```python
from build123d import *

# Parameters (mm, degrees)
F0_W      = 100.4
F0_H      = 7.3
F1_DEPTH  = 1.7
F2_R      = 1.5
F3_DEPTH  = 1.701
F4_W      = 10
F4_H      = 7.3
F5_DEPTH  = 2
F7_W      = 0.2
F7_H      = 7.3
F8_DEPTH  = 0.3
F9_W      = 0.2
F9_H      = 7.3
F10_DEPTH = 0.3


with BuildPart() as f1:
    # F0 (on Front) → F1 (new body)
    with BuildSketch(Plane.XZ):
        Rectangle(F0_W, F0_H)
    extrude(amount=F1_DEPTH)

    # F2 (on face) → F3 (cut, through all)
    with BuildSketch(Plane.XZ.offset(1.7)):
        with Locations((-28.75, -1.35)):
            Circle(F2_R)
        with Locations((-22.35, -1.35)):
            Circle(F2_R)
        with Locations((-15.95, -1.35)):
            Circle(F2_R)
        with Locations((-9.55, -1.35)):
            Circle(F2_R)
        with Locations((-3.15, -1.35)):
            Circle(F2_R)
        with Locations((3.25, -1.35)):
            Circle(F2_R)
        with Locations((9.65, -1.35)):
            Circle(F2_R)
        with Locations((16.05, -1.35)):
            Circle(F2_R)
        with Locations((22.45, -1.35)):
            Circle(F2_R)
        with Locations((28.85, -1.35)):
            Circle(F2_R)
    extrude(amount=-F3_DEPTH, mode=Mode.SUBTRACT)

    # F4 (on face) → F5 (join)
    with BuildSketch(Plane(origin=(0, 0, 0), x_dir=(-1, 0, 0), z_dir=(0, 1, 0))):
        with Locations((-45.2, 0)):
            Rectangle(F4_W, F4_H)
    extrude(amount=F5_DEPTH)

    # F7 (on face) → F8 (cut)
    with BuildSketch(Plane(origin=(0, 0, 0), x_dir=(-1, 0, 0), z_dir=(0, 1, 0))):
        with Locations((40.1, 0)):
            Rectangle(F7_W, F7_H)
    extrude(amount=-F8_DEPTH, mode=Mode.SUBTRACT)

    # F9 (on face) → F10 (cut)
    with BuildSketch(Plane(origin=(0, 0, 0), x_dir=(-1, 0, 0), z_dir=(0, 1, 0))):
        with Locations((43.1, 0)):
            Rectangle(F9_W, F9_H)
    extrude(amount=-F10_DEPTH, mode=Mode.SUBTRACT)


solid = f1.part
```
Model file for the job. Use its own axes, mm. A direction names the side the tool comes from. Give positions to 0.01 mm unless a question says otherwise; leave off trailing zeros. Loops run counter-clockwise (first coordinate to the right, second up) from the corner with the lowest first, then second, coordinate; pieces in that order, holes last. Notation, with made-up numbers: (17.25, 15) -> (53.25, 15) arc R15 cw to (53.25, 20) -> close; hole circle Ø10 at (44.25, -17). An arc over 180 degrees is marked (long way). Write each question's results on one line, items separated by ' | '.
(1) Cut at A-A on x = -9.55. List the corners of the cut face in (y, z), and give its area (3 significant figures).
Geometry results:
outline: (-1.7, -3.65) -> (0, -3.65) -> (0, -2.85) -> (-1.7, -2.85) -> close; (-1.7, 0.15) -> (0, 0.15) -> (0, 3.65) -> (-1.7, 3.65) -> close | area: 7.31 mm²
(2) Pull direction X, two halves, no side cores. Call faces 1 (the flat face through (-50.2, -1, 0)), 2 (the flat face through (-1, -1.7, 0)), 3 (the cylindrical face through (-8.744, -0.862, -0.085)): released by +X, released by -X, zero draft, split by the parting line, or undercut.
Geometry results:
face 1: released by -X | face 2: zero draft | face 3: undercut
(3) Flat gauge pins, fed straight in: pin 1 Ø2.5 at (x, z) = (16.05, -1.35) entering from -Y; pin 2 Ø3 at (x, z) = (-41, 0) entering from +Y. Where does each tip first touch, or does it go through?
Geometry results:
pin 1: passes through | pin 2: stops at y = 0
(4) Probe line 1 along Z through (x, y) = (-9.55, -0.6); line 2 along X through (y, z) = (0.3, -1.5); line 3 along Y through (x, z) = (-7.5, 2.5). List the from-to ranges inside material, lowest first.
Geometry results:
line 1: z = -3.65 to -2.85, 0.15 to 3.65 | line 2: x = 40.2 to 50.2 | line 3: y = -1.7 to 0
(5) Tool access for faces 4 (the cylindrical face through (-14.52, -0.86, -0.9)), 5 (the flat face through (-47, 0, 0)): list every direction of +Z, -Z, +X, -X, +Y, -Y with a clear straight run to the whole face (end or side of a thin tool).
Geometry results:
face 4: +Y, -Y | face 5: +Z, -Z, -X, +Y
(6) Cut at B-B on y = -0.95. Give the number of separate pieces and of enclosed holes in the cut face, and give its area (3 significant figures).
Geometry results:
separate pieces: 1 | enclosed holes: 10 | area: 662 mm²
(7) Cut at D-D on x = 18.5. List the corners of the cut face in (y, z), and give its area (3 significant figures).
Geometry results:
outline: (-1.7, -3.65) -> (0, -3.65) -> (0, 3.65) -> (-1.7, 3.65) -> close | area: 12.4 mm²
